from build123d import *

# Parameters (mm, degrees)
CROQUIS1_R              = 11
CROQUIS1_R_2            = 4
SALIENTE_EXTRUIR1_DEPTH = 7
CROQUIS2_R              = 10
CROQUIS2_R_2            = 4.5
CORTAR_EXTRUIR1_DEPTH   = 1
CORTAR_EXTRUIR2_START   = -1
CROQUIS3_R              = 10
CROQUIS3_R_2            = 4.5
CORTAR_EXTRUIR2_DEPTH   = 1


with BuildPart() as part:
    # Croquis1 → Saliente-Extruir1 (new body)
    with BuildSketch(Plane(origin=(0, 0, 0), x_dir=(0, 0, -1), z_dir=(1, 0, 0))):
        Circle(CROQUIS1_R)
        Circle(CROQUIS1_R_2, mode=Mode.SUBTRACT)
    extrude(amount=SALIENTE_EXTRUIR1_DEPTH)

    # Croquis2 → Cortar-Extruir1 (cut)
    with BuildSketch(Plane(origin=(7, 0, 0), x_dir=(0, 0, -1), z_dir=(1, 0, 0))):
        Circle(CROQUIS2_R)
        Circle(CROQUIS2_R_2, mode=Mode.SUBTRACT)
    extrude(amount=-CORTAR_EXTRUIR1_DEPTH, mode=Mode.SUBTRACT)

    # Croquis3 → Cortar-Extruir2 (cut)
    with BuildSketch(Plane.ZY.offset(CORTAR_EXTRUIR2_START)):
        with Locations(Location((0, 0, 0), (0, 0, 180))):
            Circle(CROQUIS3_R)
        with Locations(Location((0, 0, 0), (0, 0, 180))):
            Circle(CROQUIS3_R_2, mode=Mode.SUBTRACT)
    extrude(amount=CORTAR_EXTRUIR2_DEPTH, mode=Mode.SUBTRACT)


solid = part.part
The listing builds one solid part. Answer for the finished solid, in the listing's coordinates (mm). A direction names the side the tool comes from. Give positions to 0.01 mm unless a question says otherwise; leave off trailing zeros. Order: outer loops, then holes, each group sorted by start corner. A loop starts at its lowest first (then second) coordinate and runs counter-clockwise, first axis right, second up. Notation, with made-up numbers: (63, -10.5) - (85, -10.5) arc R24 cw to (85, 5.5) - close; hole circle Ø4 at (49.5, -3). An arc over 180 degrees is marked (long way). Use one line per item in the form item = value.
1) Each of these flat-tipped pins is pushed along its axis until it touches: pin 1 (3 mm diameter, centred on x = 4, z = 7.5, fed in from -Y); pin 2 (2 mm diameter, centred on x = 4.5, y = -1.5, fed in from -Z); pin 3 (1.5 mm diameter, centred on x = 1, z = 5.5, fed in from +Y). Where does it stop, or does it pass through?
Verdict:
pin_1 = -9.22
pin_2 = -10.99
pin_3 = 9.92
2) Find section D-D on y = 7.5. Determine the outline of the cut face in (x, z), and give its area (3 significant figures).
Verdict:
outline = (0, -8.05) - (7, -8.05) - (7, -6.61) - (6, -6.61) - (6, 6.61) - (7, 6.61) - (7, 8.05) - (0, 8.05) - (0, 6.61) - (1, 6.61) - (1, -6.61) - (0, -6.61) - close
area = 86.2 mm^2
3) For faces 1 (the cylindrical face through (0.51, -3.04, 3.32)), 2 (the flat face through (0, -3, 3)), 3 (the cylindrical face through (6.51, -9.76, 2.17)), determine the directions among +Z, -Z, +X, -X, +Y, -Y from which every point of the face is accessible in a straight line to the end or side of a thin tool.
Verdict:
face_1 = -X
face_2 = +Z, -Z, -X, +Y, -Y
face_3 = +X
4) Find section C-C on x = 3. Determine the outline of the cut face in (y, z), and give its area (3 significant figures).
Verdict:
outline = circle Ø22 at (0, 0); hole circle Ø8 at (0, 0)
area = 330 mm^2
5) Consider probe 1 along Y at (x, z) = (0.6, 0); probe 2 along Y at (x, z) = (6.5, 3); probe 3 along Y at (x, z) = (1.5, 0). Determine where each line is inside the solid, lowest interval first. Write a range as [from, to].
Verdict:
probe_1 = [-11, -10], [-4.5, -4], [4, 4.5], [10, 11]
probe_2 = [-10.58, -9.54], [-3.35, -2.65], [2.65, 3.35], [9.54, 10.58]
probe_3 = [-11, -4], [4, 11]
6) The mould has two halves that part along Z. Classify faces 4 (the cylindrical face through (6.51, 4.46, 0.59)), 5 (the cylindrical face through (3.45, -10.74, 2.38)), 6 (the flat face through (7, -3, 3)): released by +Z, released by -Z, zero draft, split by the parting line, or undercut.
Verdict:
face_4 = undercut
face_5 = split by the parting line
face_6 = zero draft
7) Find section A-A on z = 0. Determine the outline of the cut face in (x, y).
Verdict:
outline = (0, -11) - (7, -11) - (7, -10) - (6, -10) - (6, -4.5) - (7, -4.5) - (7, -4) - (0, -4) - (0, -4.5) - (1, -4.5) - (1, -10) - (0, -10) - close; (0, 4) - (7, 4) - (7, 4.5) - (6, 4.5) - (6, 10) - (7, 10) - (7, 11) - (0, 11) - (0, 10) - (1, 10) - (1, 4.5) - (0, 4.5) - close
